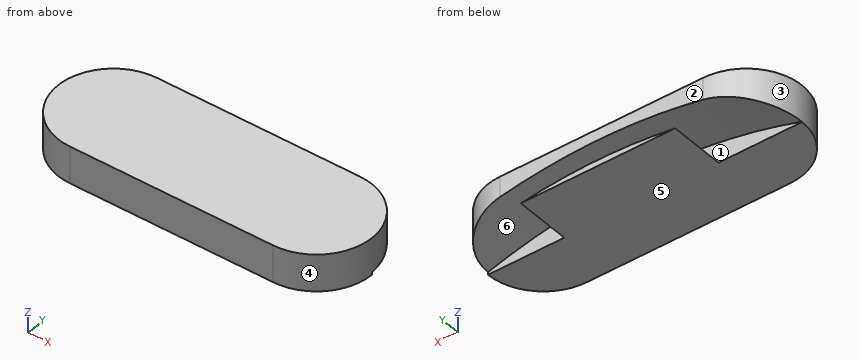
```python
from build123d import *

# Parameters (mm, degrees)
F1_DEPTH = 12.7
F3_DEPTH = 50.8


with BuildPart() as f1:
    # F0 (on Top) → F1 (new body)
    with BuildSketch(Plane.XY):
        with BuildLine():
            ThreePointArc((34.924999, -19.05), (53.974999, -1e-06), (34.925001, 19.05))
            Line((34.925001, 19.05), (-34.924999, 19.05))
            ThreePointArc((-34.924999, 19.05), (-53.975001, 1e-06), (-34.925001, -19.05))
            Line((-34.925001, -19.05), (34.924999, -19.05))
        make_face()
    extrude(amount=F1_DEPTH)

    # F2 (on Front) → F3 (cut)
    with BuildSketch(Plane.XZ):
        with BuildLine():
            ThreePointArc((-25.293126, 0), (1.228994, 2.061294), (27.751113, 0))
            Line((27.751113, 0), (56.808557, 0))
            ThreePointArc((56.808557, 0), (1.228994, 8.874986), (-54.35057, 0))
            Line((-54.35057, 0), (-25.293126, 0))
        make_face()
    extrude(amount=-F3_DEPTH, mode=Mode.SUBTRACT)


solid = f1.part
```
Geometry: final body of the model. Coordinates: model frame, mm. Face numbers are marked on the shaded views. A direction names the side the tool comes from. Coordinates: 2 decimals unless noted, no trailing zeros. Loops run counter-clockwise (first coordinate to the right, second up) from the corner with the lowest first, then second, coordinate; pieces in that order, holes last. Notation, with made-up numbers: (67, 80.25) -> (107, 80.25) arc R18 ccw to (107, 87.25) -> close; hole circle Ø1 at (66.5, -5.75). An arc over 180 degrees is marked (long way). Use a Markdown table: item, result. Add a question column.
(1) Mould query, pull axis X, two halves, no side actions, for the marked faces 1, 2, 3 and 4. Classes: pulls with the +X half, pulls with the -X half, needs draft (parallel to the pull), parting line crosses it, or undercut.
(2) Section query D-D, the plane y = 11.5. Return loops of the section in (x, z), plus the area to 3 significant figures.
(3) Section query A-A, the plane y = 17. Return loops of the section in (x, z).
(4) Pin query (flat end, axial travel): pin 1 Ø4.5 at (x, z) = (-6, 3.5) entering from +Y; pin 2 Ø2 at (y, z) = (-3.5, 2.5) entering from -X; pin 3 Ø1.5 at (y, z) = (-6.5, 8.5) entering from -X; pin 4 Ø1 at (x, y) = (34.5, 11) entering from -Z. Return the tip coordinate at first contact, or that it passes through.
(5) Section query B-B, the plane z = 11.75. Return loops of the section in (x, y) (3 decimals).
(6) Access query for the marked faces 5 and 6. Directions: +Z, -Z, +X, -X, +Y, -Y. A direction counts if a zero-diameter tool reaches every point of the face in a straight line with its end or side. Return the directions, or none.
(7) Section query C-C, the plane x = -5. Return loops of the section in (y, z), plus the area to 3 significant figures.
(8) Line query: line 1 along Y through (x, z) = (16, 5.25); line 2 along Z through (x, y) = (-11.5, 6.5); line 3 along Z through (x, y) = (-4, 17). Output: solid intervals per line, ascending.
Answer:
| question | item | result |
|---|---|---|
| 1 | face 1 | undercut |
| 1 | face 2 | needs draft |
| 1 | face 3 | pulls with the -X half |
| 1 | face 4 | pulls with the +X half |
| 2 | outline | (-50.11, 1.33) arc R178.47 cw to (50.11, 2.05) -> (50.11, 12.7) -> (-50.11, 12.7) -> close; (-25.29, 0) -> (27.75, 0) arc R171.66 ccw to start |
| 2 | area | 695 mm^2 |
| 3 | outline | (-43.52, 3.17) arc R178.47 cw to (43.52, 3.79) -> (43.52, 12.7) -> (-43.52, 12.7) -> close; (-25.29, 0) -> (27.75, 0) arc R171.66 ccw to start |
| 4 | pin 1 | stops at y = 19.05 |
| 4 | pin 2 | stops at x = -53.81 |
| 4 | pin 3 | stops at x = -53.09 |
| 4 | pin 4 | stops at z = 5.65 |
| 5 | outline | (-34.925, -19.05) -> (34.925, -19.05) arc R19.05 ccw to (34.925, 19.05) -> (-34.925, 19.05) arc R19.05 ccw to start |
| 6 | face 5 | -Z, +X, -X, +Y, -Y |
| 6 | face 6 | +Y |
| 7 | outline | (-19.05, 0) -> (19.05, 0) -> (19.05, 1.95) -> (0, 1.95) -> (0, 8.77) -> (19.05, 8.77) -> (19.05, 12.7) -> (-19.05, 12.7) -> close |
| 7 | area | 354 mm^2 |
| 8 | line 1 | y = -19.05 to 0 |
| 8 | line 2 | z = 0 to 1.59, 8.42 to 12.7 |
| 8 | line 3 | z = 0 to 1.98, 8.8 to 12.7 |
